Read the model definition and answer for the solid it produces. Units are mm, in the model's axes. A direction names the side the tool comes from. Round coordinates to 2 decimals unless told otherwise and drop trailing zeros. Write each loop counter-clockwise with the first axis right and the second up, starting at its lowest first coordinate (ties: lowest second). Pieces come first, ordered by that corner, then holes. Notation, with made-up numbers: (54, -20.75) - (100, -20.75) arc R17 ccw to (100, -12.75) - close; hole circle Ø9 at (87.5, 70.5). An arc over 180 degrees is marked (long way). One line per item, written item: value. Start each with the question number.
(1) A cutting plane is placed at A-A, the plane y = 0. Determine the outline of the cut face in (x, z).
(2) A cutting plane is placed at C-C, the plane z = -133. Determine the outline of the cut face in (x, y).
(3) A cutting plane is placed at B-B, the plane x = 29.5. Determine the outline of the cut face in (y, z), plus the area to 3 significant figures.
(4) For faces 1 (the face through (20, 4, -360)), 2 (the face through (0, 0, 0)), 3 (the face through (-6, 0, -185)), 4 (the face through (20, -4, -360)), determine the directions among +Z, -Z, +X, -X, +Y, -Y from which every point of the face is accessible in a straight line to the end or side of a thin tool.
(5) Find the intervals of material crossed by L1, parallel to Z at x = 6, y = -3; L2, parallel to Y at x = 19, z = -359.5; L3, parallel to X at y = 4.5, z = -36, in increasing order.
(6) Flat-ended cylindrical pins translate along their axes: pin 1 Ø24 at (x, z) = (20, -366.5) entering from +Y; pin 2 Ø4 at (x, z) = (5, -318.5) entering from -Y; pin 3 Ø2.5 at (x, y) = (13, -0.5) entering from +Z. Find the tip coordinate at first contact, or state that the pin passes through.
from build123d import *

# Parameters (mm, degrees)
SKETCH1_R           = 6
BOSS_EXTRUDE1_DEPTH = 375
SKETCH2_W           = 30
SKETCH2_H           = 8
BOSS_EXTRUDE2_DEPTH = 35


with BuildPart() as part:
    # Sketch1 → Boss-Extrude1 (new body)
    with BuildSketch(Plane.XY):
        Circle(SKETCH1_R)
    extrude(amount=-BOSS_EXTRUDE1_DEPTH)

    # Sketch2 → Boss-Extrude2 (add)
    with BuildSketch(Plane(origin=(0, 0, 0), x_dir=(0, 0, -1), z_dir=(1, 0, 0))):
        with Locations((360, 0)):
            Rectangle(SKETCH2_W, SKETCH2_H)
    extrude(amount=BOSS_EXTRUDE2_DEPTH)


solid = part.part
Here are the results:
1. outline: (-6, -375) - (35, -375) - (35, -345) - (6, -345) - (6, 0) - (-6, 0) - close
2. outline: circle Ø12 at (0, 0)
3. outline: (-4, -375) - (4, -375) - (4, -345) - (-4, -345) - close
3. area: 240 mm²
4. face 1: +Z, -Z, +X, +Y
4. face 2: +Z, +X, -X, +Y, -Y
4. face 3: +Z
4. face 4: +Z, -Z, +X, -Y
5. L1: -375 to -345
5. L2: -4 to 4
5. L3: -3.97 to 3.97
6. pin 1: y = 4
6. pin 2: y = -5.2
6. pin 3: z = -345
